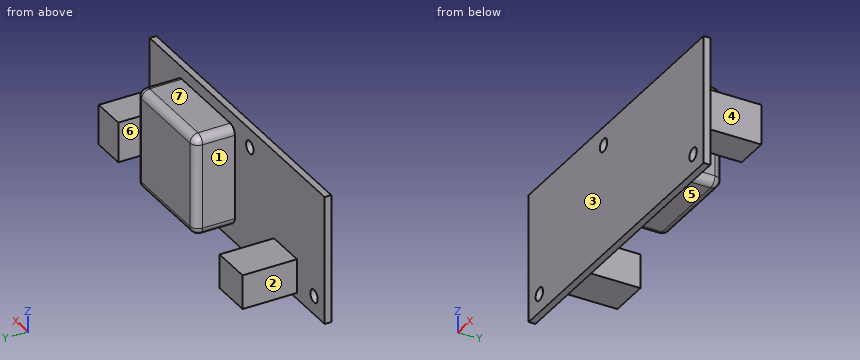
```python
from build123d import *

# Parameters (mm, degrees)
SKETCH1_W                = 76
SKETCH1_H                = 32
BOSS_EXTRUDE1_DEPTH      = 1.65
M3_CLEARANCE_HOLE1_D     = 3.2
M3_CLEARANCE_HOLE1_DEPTH = 20
M3_CLEARANCE_HOLE1_TIP   = 0.96137699
SKETCH4_W                = 10
SKETCH4_H                = 8.5
SKETCH4_W_2              = 8.5
SKETCH4_H_2              = 10
BOSS_EXTRUDE2_DEPTH      = 13.5
SKETCH5_W                = 25
SKETCH5_H                = 25
BOSS_EXTRUDE3_DEPTH      = 10
FILLET1_R                = 2


with BuildPart() as part:
    # Sketch1 → Boss-Extrude1 (new body)
    with BuildSketch(Plane(origin=(0, 0, 0), x_dir=(1, 0, 0), z_dir=(0, 1, 0))):
        with Locations((38, 16)):
            Rectangle(SKETCH1_W, SKETCH1_H)
    extrude(amount=BOSS_EXTRUDE1_DEPTH)

    # M3 Clearance Hole1
    with Locations(Plane(origin=(0, 1.65, 0), x_dir=(1, 0, 0), z_dir=(0, 1, 0))):
        with Locations((71.4, 27.4), (32.5, 4.6), (4.6, 27.4)):
            Hole(M3_CLEARANCE_HOLE1_D / 2, depth=M3_CLEARANCE_HOLE1_DEPTH)
            with Locations((0, 0, -(M3_CLEARANCE_HOLE1_DEPTH + M3_CLEARANCE_HOLE1_TIP / 2))):  # 118° drill point
                Cone(0, M3_CLEARANCE_HOLE1_D / 2, M3_CLEARANCE_HOLE1_TIP, mode=Mode.SUBTRACT)

    # Sketch4 → Boss-Extrude2 (add)
    with BuildSketch(Plane(origin=(0, 1.65, 0), x_dir=(1, 0, 0), z_dir=(0, 1, 0))):
        with Locations((17, 26.25)):
            Rectangle(SKETCH4_W, SKETCH4_H)
        with Locations((70.25, 17)):
            Rectangle(SKETCH4_W_2, SKETCH4_H_2)
    extrude(amount=BOSS_EXTRUDE2_DEPTH)

    # Sketch5 → Boss-Extrude3 (add)
    with BuildSketch(Plane(origin=(0, 1.65, 0), x_dir=(1, 0, 0), z_dir=(0, 1, 0))):
        with Locations((51.5, 15.5)):
            Rectangle(SKETCH5_W, SKETCH5_H)
    extrude(amount=BOSS_EXTRUDE3_DEPTH)

    # Fillet1
    fillet1_edges = [part.edges().sort_by_distance(p)[0] for p in [
        (64, 6.65, -3),
        (64, 6.65, -28),
        (39, 6.65, -28),
        (39, 6.65, -3),
        (64, 11.65, -15.5),
        (51.5, 11.65, -28),
        (39, 11.65, -15.5),
        (51.5, 11.65, -3),
    ]]
    fillet(fillet1_edges, radius=FILLET1_R)


solid = part.part
```
Geometry check sheet. Reference: the model listing, model coordinates, mm. Face numbers are marked on the shaded views. A direction names the side the tool comes from. Coordinates: 2 decimals unless noted, no trailing zeros. Loops run counter-clockwise (first coordinate to the right, second up) from the corner with the lowest first, then second, coordinate; pieces in that order, holes last.
Item 1: Sectioned sample at C-C, the plane z = -25. Record the boundary of the cut face in (x, y).
Item 2: Sectioned sample at D-D, the plane x = 4.6. Record the boundary of the cut face in (y, z), then the cut area to 3 significant figures.
Item 3: Sectioned sample at A-A, the plane y = 5.5. Record the boundary of the cut face in (x, z).
Item 4: Release check for a two-part mould opening along X. For the marked faces 1, 2, 3 and 4 record: released by +X, released by -X, zero draft, split by the parting line, or undercut.
Item 5: Thickness scan on line 1 (X direction, y = 0.5, z = -27.4); line 2 (X direction, y = 1.2, z = -4.6); line 3 (X direction, y = 4, z = -16). Record the ranges inside material, lowest first.
Item 6: Access from +Z, -Z, +X, -X, +Y, -Y to the whole of each face (thin tool, end or side, straight path). Record for the marked faces 5, 6 and 7.
Item 7: Sectioned sample at B-B, the plane x = 71.4. Record the boundary of the cut face in (y, z).
Item 8: Go/stop test with flat-tipped pins: pin 1 Ø5 at (x, z) = (32.5, -4.6) entering from +Y; pin 2 Ø7 at (y, z) = (7, -26.5) entering from +X; pin 3 Ø6.5 at (y, z) = (7.5, -13) entering from -X. Record where each tip stops, or that it passes through.
Check result:
1. outline: (0, 0) - (76, 0) - (76, 1.65) - (64, 1.65) - (64, 9.65) arc R2 ccw to (62, 11.65) - (41, 11.65) arc R2 ccw to (39, 9.65) - (39, 1.65) - (22, 1.65) - (22, 15.15) - (12, 15.15) - (12, 1.65) - (0, 1.65) - close
2. outline: (0, -32) - (1.65, -32) - (1.65, -29) - (0, -29) - close; (0, -25.8) - (1.65, -25.8) - (1.65, 0) - (0, 0) - close
2. area: 47.5 mm2
3. outline: (12, -30.5) - (22, -30.5) - (22, -22) - (12, -22) - close; (39, -26) arc R2 ccw to (41, -28) - (62, -28) arc R2 ccw to (64, -26) - (64, -5) arc R2 ccw to (62, -3) - (41, -3) arc R2 ccw to (39, -5) - close; (66, -22) - (74.5, -22) - (74.5, -12) - (66, -12) - close
4. face 1: undercut
4. face 2: released by -X
4. face 3: zero draft
4. face 4: released by +X
5. line 1: x = 0 to 3, 6.2 to 69.8, 73 to 76
5. line 2: x = 0 to 30.9, 34.1 to 76
5. line 3: x = 39 to 64, 66 to 74.5
6. face 5: -Z, +X, +Y
6. face 6: +Z, -Z, +Y
6. face 7: +Z, +X, -X, +Y
7. outline: (0, -32) - (1.65, -32) - (1.65, -29) - (0, -29) - close; (0, -25.8) - (1.65, -25.8) - (1.65, -22) - (15.15, -22) - (15.15, -12) - (1.65, -12) - (1.65, 0) - (0, 0) - close
8. pin 1: stops at y = 1.65
8. pin 2: stops at x = 64
8. pin 3: stops at x = 39
